Build history of the part. All positions in model axes, mm. A direction names the side the tool comes from. Give positions to 0.01 mm unless a question says otherwise; leave off trailing zeros. Write each loop counter-clockwise with the first axis right and the second up, starting at its lowest first coordinate (ties: lowest second). Pieces come first, ordered by that corner, then holes.
from build123d import *

# Parameters (mm, degrees)
BASE_FLANGE1_DEPTH = 1215
SKETCH6_W          = 110
SKETCH6_H          = 6
CUT_EXTRUDE1_DEPTH = 1257.7008395
CUT_EXTRUDE2_DEPTH = 1257.7008395
SKETCH8_R          = 6
CUT_EXTRUDE3_DEPTH = 1257.357035241
FILLET1_R          = 10


# Sheet-metal steps are written as plain solids
with BuildPart() as part:
    # Sketch1 → Base-Flange1 (new body)
    with BuildSketch(Plane.XY):
        with BuildLine():
            Line((-40, 164), (-6, 164))
            ThreePointArc((-6, 164), (-1.757359313, 162.242640687), (0, 158))
            Line((0, 158), (0, 2))
            ThreePointArc((0, 2), (0.585786438, 0.585786438), (2, 0))
            Line((2, 0), (230, 0))
            ThreePointArc((230, 0), (231.414213562, 0.585786438), (232, 2))
            Line((232, 2), (232, 158))
            ThreePointArc((232, 158), (233.757359313, 162.242640687), (238, 164))
            Line((238, 164), (272, 164))
            Line((272, 164), (272, 160))
            Line((272, 160), (238, 160))
            ThreePointArc((238, 160), (236.585786438, 159.414213562), (236, 158))
            Line((236, 158), (236, 2))
            ThreePointArc((236, 2), (234.242640687, -2.242640687), (230, -4))
            Line((230, -4), (2, -4))
            ThreePointArc((2, -4), (-2.242640687, -2.242640687), (-4, 2))
            Line((-4, 2), (-4, 158))
            ThreePointArc((-4, 158), (-4.585786438, 159.414213562), (-6, 160))
            Line((-6, 160), (-40, 160))
            Line((-40, 160), (-40, 164))
        make_face()
    extrude(amount=BASE_FLANGE1_DEPTH)

    # Sketch6 → Cut-Extrude1 (cut, through all)
    with BuildSketch(Plane(origin=(-4, 0, 0), x_dir=(0, 0, -1), z_dir=(1, 0, 0))):
        with Locations((-55, -1)):
            Rectangle(SKETCH6_W, SKETCH6_H)
        with Locations((-1160, -1)):
            Rectangle(SKETCH6_W, SKETCH6_H)
    extrude(amount=CUT_EXTRUDE1_DEPTH, mode=Mode.SUBTRACT)

    # Sketch7 → Cut-Extrude2 (cut, through all)
    with BuildSketch(Plane.ZY.offset(4)):
        with BuildLine():
            Line((26, 119), (16, 119))
            ThreePointArc((16, 119), (9, 126), (16, 133))
            Line((16, 133), (26, 133))
            ThreePointArc((26, 133), (33, 126), (26, 119))
        make_face()
        with BuildLine():
            Line((71, 119), (61, 119))
            ThreePointArc((61, 119), (54, 126), (61, 133))
            Line((61, 133), (71, 133))
            ThreePointArc((71, 133), (78, 126), (71, 119))
        make_face()
        with BuildLine():
            Line((71, 74), (61, 74))
            ThreePointArc((61, 74), (54, 81), (61, 88))
            Line((61, 88), (71, 88))
            ThreePointArc((71, 88), (78, 81), (71, 74))
        make_face()
        with BuildLine():
            Line((71, 29), (61, 29))
            ThreePointArc((61, 29), (54, 36), (61, 43))
            Line((61, 43), (71, 43))
            ThreePointArc((71, 43), (78, 36), (71, 29))
        make_face()
        with BuildLine():
            Line((26, 74), (16, 74))
            ThreePointArc((16, 74), (9, 81), (16, 88))
            Line((16, 88), (26, 88))
            ThreePointArc((26, 88), (33, 81), (26, 74))
        make_face()
        with BuildLine():
            Line((26, 29), (16, 29))
            ThreePointArc((16, 29), (9, 36), (16, 43))
            Line((16, 43), (26, 43))
            ThreePointArc((26, 43), (33, 36), (26, 29))
        make_face()
        with BuildLine():
            Line((1189, 119), (1199, 119))
            ThreePointArc((1199, 119), (1206, 126), (1199, 133))
            Line((1199, 133), (1189, 133))
            ThreePointArc((1189, 133), (1182, 126), (1189, 119))
        make_face()
        with BuildLine():
            Line((1144, 119), (1154, 119))
            ThreePointArc((1154, 119), (1161, 126), (1154, 133))
            Line((1154, 133), (1144, 133))
            ThreePointArc((1144, 133), (1137, 126), (1144, 119))
        make_face()
        with BuildLine():
            Line((1144, 74), (1154, 74))
            ThreePointArc((1154, 74), (1161, 81), (1154, 88))
            Line((1154, 88), (1144, 88))
            ThreePointArc((1144, 88), (1137, 81), (1144, 74))
        make_face()
        with BuildLine():
            Line((1144, 29), (1154, 29))
            ThreePointArc((1154, 29), (1161, 36), (1154, 43))
            Line((1154, 43), (1144, 43))
            ThreePointArc((1144, 43), (1137, 36), (1144, 29))
        make_face()
        with BuildLine():
            Line((1189, 74), (1199, 74))
            ThreePointArc((1199, 74), (1206, 81), (1199, 88))
            Line((1199, 88), (1189, 88))
            ThreePointArc((1189, 88), (1182, 81), (1189, 74))
        make_face()
        with BuildLine():
            Line((1189, 29), (1199, 29))
            ThreePointArc((1199, 29), (1206, 36), (1199, 43))
            Line((1199, 43), (1189, 43))
            ThreePointArc((1189, 43), (1182, 36), (1189, 29))
        make_face()
    extrude(amount=-CUT_EXTRUDE2_DEPTH, mode=Mode.SUBTRACT)

    # Sketch8 → Cut-Extrude3 (cut, through all)
    with BuildSketch(Plane(origin=(0, 164, 0), x_dir=(1, 0, 0), z_dir=(0, 1, 0))):
        with Locations(Location((116, -607.5, 0), (0, 0, 270))):
            Circle(SKETCH8_R)
        with BuildLine():
            Line((249, -1149.5), (249, -1064.5))
            ThreePointArc((249, -1064.5), (256, -1057.5), (263, -1064.5))
            Line((263, -1064.5), (263, -1149.5))
            ThreePointArc((263, -1149.5), (256, -1156.5), (249, -1149.5))
        make_face()
        with BuildLine():
            Line((249, -65.5), (249, -150.5))
            ThreePointArc((249, -150.5), (256, -157.5), (263, -150.5))
            Line((263, -150.5), (263, -65.5))
            ThreePointArc((263, -65.5), (256, -58.5), (249, -65.5))
        make_face()
        with BuildLine():
            Line((-17, -65.5), (-17, -150.5))
            ThreePointArc((-17, -150.5), (-24, -157.5), (-31, -150.5))
            Line((-31, -150.5), (-31, -65.5))
            ThreePointArc((-31, -65.5), (-24, -58.5), (-17, -65.5))
        make_face()
        with BuildLine():
            Line((-17, -1149.5), (-17, -1064.5))
            ThreePointArc((-17, -1064.5), (-24, -1057.5), (-31, -1064.5))
            Line((-31, -1064.5), (-31, -1149.5))
            ThreePointArc((-31, -1149.5), (-24, -1156.5), (-17, -1149.5))
        make_face()
    extrude(amount=-CUT_EXTRUDE3_DEPTH, mode=Mode.SUBTRACT)

    # Fillet1
    fillet1_edges = [part.edges().sort_by_distance(p)[0] for p in [
        (234, 2, 0),
        (234, 2, 1215),
        (-2, 2, 0),
        (-2, 2, 1215),
    ]]
    fillet(fillet1_edges, radius=FILLET1_R)


solid = part.part
1. Drop flat-ended pins along their axis: pin 1 (3 mm diameter, centred on x = 233, z = 1148.5, fed in from +Y); pin 2 (4 mm diameter, centred on y = 50.5, z = 240, fed in from +X); pin 3 (2 mm diameter, centred on x = 233.5, z = 1196.5, fed in from -Y); pin 4 (11 mm diameter, centred on x = 116, z = 607.5, fed in from +Y). Give the stop position or say it passes through.
2. Saw through at B-B on x = 202. Give the cut face in (y, z), plus the area to 3 significant figures.
3. Drill centre lines: line 1 along X through (y, z) = (14, 927.5); line 2 along Y through (x, z) = (132, 610); line 3 along X through (y, z) = (-0.95, 607.5). Where is each one in solid material? Low to high.
4. Mould opens along X. For faces 1 (the face through (236, 81, 599)), 2 (the face through (235.8, 105.2, 1215)), 3 (the face through (114, 0, 601)) say: pulls with the +X half, pulls with the -X half, needs draft (parallel to the pull), parting line crosses it, or undercut.
5. Saw through at A-A on z = 396. Give the cut face in (x, y), plus the area to 3 significant figures.
6. 3-axis set-ups, long thin cutter, end or side, ignore diameter. For faces 4 (the face through (0, 81, 599)), 5 (the face through (-23, 160, 599)), 6 (the face through (255, 160, 599)): which of +Z, -Z, +X, -X, +Y, -Y reach the whole face in a straight line?
Outcome:
1. pin 1: stops at y = 162.87
1. pin 2: stops at x = 236
1. pin 3: stops at y = 2
1. pin 4: passes through
2. outline: (-4, 110) - (0, 110) - (0, 1105) - (-4, 1105) - close
2. area: 3,980 mm2
3. line 1: x = -4 to 0, 232 to 236
3. line 2: y = -4 to 0
3. line 3: x = -3.22 to 110, 122 to 235.22
4. face 1: pulls with the +X half
4. face 2: needs draft
4. face 3: undercut
5. outline: (-40, 160) - (-6, 160) arc R2 cw to (-4, 158) - (-4, 2) arc R6 ccw to (2, -4) - (230, -4) arc R6 ccw to (236, 2) - (236, 158) arc R2 cw to (238, 160) - (272, 160) - (272, 164) - (238, 164) arc R6 ccw to (232, 158) - (232, 2) arc R2 cw to (230, 0) - (2, 0) arc R2 cw to (0, 2) - (0, 158) arc R6 ccw to (-6, 164) - (-40, 164) - close
5. area: 2,530 mm2
6. face 4: +Z, -Z, +Y
6. face 5: +Z, -Z, -X, -Y
6. face 6: +Z, -Z, +X, -Y
